Job drawing, mm, ordinate dimensions from the low corner. One solid piece. A direction names the side the tool comes from. Coordinates: 2 decimals unless noted, no trailing zeros. Order: outer loops, then holes, each group sorted by start corner. A loop starts at its lowest first (then second) coordinate and runs counter-clockwise, first axis right, second up. Notation, with made-up numbers: (2, -35) -> (30, -35) arc R19 cw to (30, -9) -> close; hole circle Ø4 at (47.5, -21.5). An arc over 180 degrees is marked (long way). Use CSV: the item, a comma, the result in double quotes. Start each with the question number.
(1) Tool access for the marked faces 1, 2 and 3: list every direction of +Z, -Z, +X, -X, +Y, -Y with a clear straight run to the whole face (end or side of a thin tool).
(2) Pull direction X, two halves, no side cores. Call the marked faces 4, 5 and 6: pulls with the +X half, pulls with the -X half, needs draft (parallel to the pull), parting line crosses it, or undercut.
(3) Cut at A-A on z = 47. Write the cut outline in (x, y) (3 decimals).
(4) Probe L1, parallel to X at y = 89, z = 45 (3 decimals); L2, parallel to Y at x = 14, z = 25.5 (3 decimals). List the from-to ranges inside material, lowest first.
(5) Pin check, flat tips, straight feed: pin 1 Ø10 at (x, z) = (46, 44) entering from +Y; pin 2 Ø6.5 at (y, z) = (88, 42) entering from -X; pin 3 Ø10 at (y, z) = (41.5, 46) entering from +X. Stop position of each tip, or through.
(6) Cut at B-B on x = 84. Write the cut outline in (y, z) (3 decimals).
(7) Cut at D-D on z = 24.5. Write the cut outline in (x, y) (3 decimals).
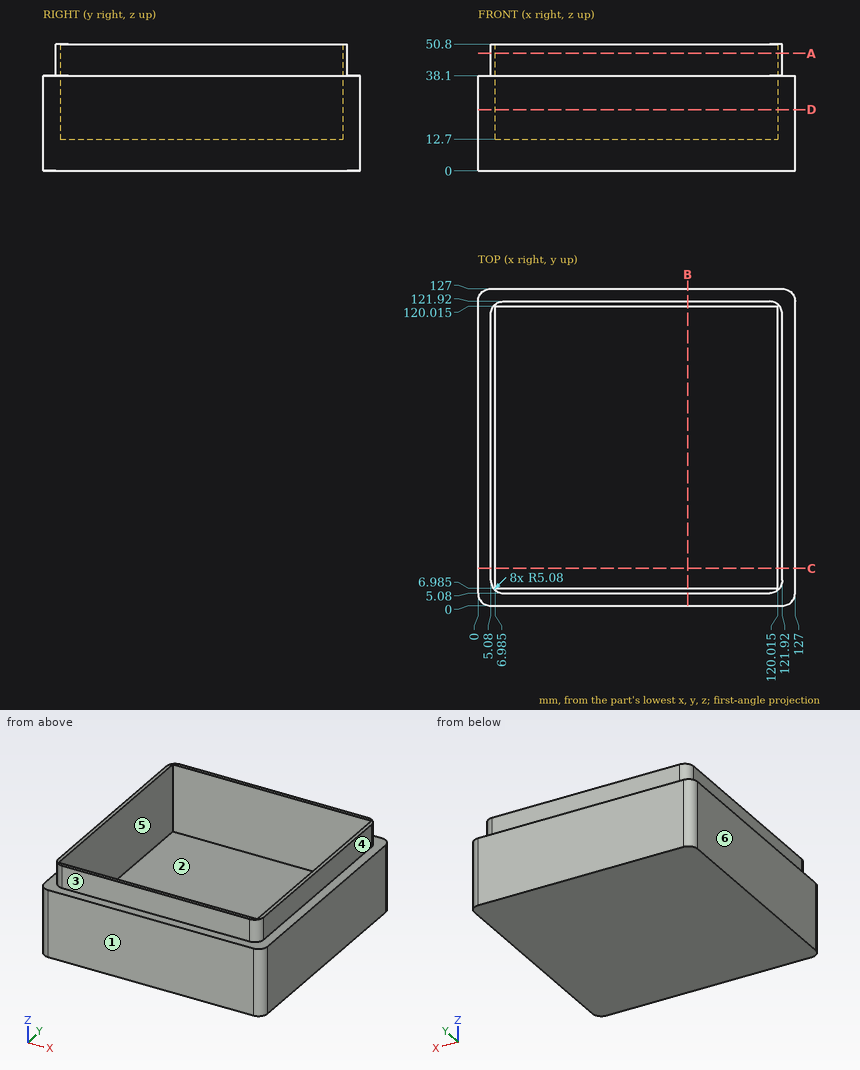
Outcome:
1,face 1,"+Z, -Z, +X, -X, -Y"
1,face 2,"+Z"
1,face 3,"+Z, +X, -X, -Y"
2,face 4,"pulls with the +X half"
2,face 5,"undercut"
2,face 6,"pulls with the -X half"
3,outline,"(5.08, 10.16) arc R5.08 ccw to (10.16, 5.08) -> (116.84, 5.08) arc R5.08 ccw to (121.92, 10.16) -> (121.92, 116.84) arc R5.08 ccw to (116.84, 121.92) -> (10.16, 121.92) arc R5.08 ccw to (5.08, 116.84) -> close; hole (6.985, 6.985) -> (120.015, 6.985) -> (120.015, 120.015) -> (6.985, 120.015) -> close"
4,L1,"5.08 to 6.985, 120.015 to 121.92"
4,L2,"0 to 6.985, 120.015 to 127"
5,pin 1,"y = 121.92"
5,pin 2,"x = 5.08"
5,pin 3,"x = 121.92"
6,outline,"(0, 0) -> (127, 0) -> (127, 38.1) -> (121.92, 38.1) -> (121.92, 50.8) -> (120.015, 50.8) -> (120.015, 12.7) -> (6.985, 12.7) -> (6.985, 50.8) -> (5.08, 50.8) -> (5.08, 38.1) -> (0, 38.1) -> close"
7,outline,"(0, 5.08) arc R5.08 ccw to (5.08, 0) -> (121.92, 0) arc R5.08 ccw to (127, 5.08) -> (127, 121.92) arc R5.08 ccw to (121.92, 127) -> (5.08, 127) arc R5.08 ccw to (0, 121.92) -> close; hole (6.985, 6.985) -> (120.015, 6.985) -> (120.015, 120.015) -> (6.985, 120.015) -> close"
